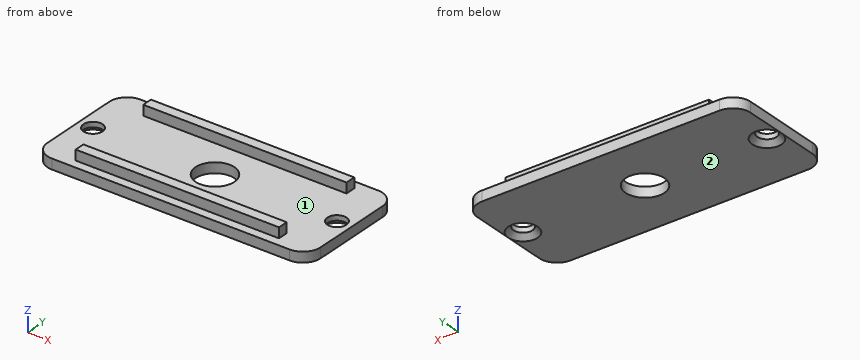
```python
from build123d import *

# Parameters (mm, degrees)
F1_DEPTH = 2
F2_R     = 1.875
F3_DEPTH = 2.001
F4_SIZE  = 0.99999
F5_W     = 40
F5_H     = 2
F6_DEPTH = 2
F7_R     = 3.81
F8_DEPTH = 2.001


# Not quite as in the source:
# - a fillet or chamfer is up to 0.001 mm smaller than in the source, because OpenCascade refuses the exact size


with BuildPart() as f1:
    # F0 (on Top) → F1 (new body)
    with BuildSketch(Plane.XY):
        with BuildLine():
            ThreePointArc((26.875, 8), (25.8498737342, 10.4748737342), (23.375, 11.5))
            Line((23.375, 11.5), (-23.375, 11.5))
            ThreePointArc((-23.375, 11.5), (-25.8498737342, 10.4748737342), (-26.875, 8))
            Line((-26.875, 8), (-26.875, -8))
            ThreePointArc((-26.875, -8), (-25.8498737342, -10.4748737342), (-23.375, -11.5))
            Line((-23.375, -11.5), (23.375, -11.5))
            ThreePointArc((23.375, -11.5), (25.8498737342, -10.4748737342), (26.875, -8))
            Line((26.875, -8), (26.875, 8))
        make_face()
    extrude(amount=F1_DEPTH)

    # F2 (on face) → F3 (cut, through all)
    with BuildSketch(Plane.XY.offset(2)):
        with Locations((-24, 0)):
            Circle(F2_R)
        with Locations((24, 0)):
            Circle(F2_R)
    extrude(amount=-F3_DEPTH, mode=Mode.SUBTRACT)

    # F4 (size 1 in the source; OpenCascade refuses exactly that, so slightly less here)
    f4_edges = [f1.edges().sort_by_distance(p)[0] for p in [
        (-25.875, 0, 0),
        (22.125, 0, 0),
    ]]
    chamfer(f4_edges, length=F4_SIZE)

    # F5 (on face) → F6 (join)
    with BuildSketch(Plane.XY.offset(2)):
        with Locations((0, 8.75)):
            Rectangle(F5_W, F5_H)
        with Locations((0, -8.75)):
            Rectangle(F5_W, F5_H)
    extrude(amount=F6_DEPTH)

    # F7 (on face) → F8 (cut, through all)
    with BuildSketch(Plane.XY.offset(2)):
        Circle(F7_R)
    extrude(amount=-F8_DEPTH, mode=Mode.SUBTRACT)


solid = f1.part
```
For this review, take the finished solid that the model builds, in its own axes (mm). Face numbers are marked on the shaded views. Round coordinates to 2 decimals unless told otherwise and drop trailing zeros. Loops run counter-clockwise (first coordinate to the right, second up) from the corner with the lowest first, then second, coordinate; pieces in that order, holes last.
(1) We need section C-C (x = -19). Give the boundary of the cut face in (y, z).
Returned:
outline: (-11.5, 0) - (11.5, 0) - (11.5, 2) - (9.75, 2) - (9.75, 4) - (7.75, 4) - (7.75, 2) - (-7.75, 2) - (-7.75, 4) - (-9.75, 4) - (-9.75, 2) - (-11.5, 2) - close
(2) We need section D-D (x = 24). Give the boundary of the cut face in (y, z) (3 decimals), plus the area to 3 significant figures.
Returned:
outline: (-11.444, 0) - (-2.875, 0) - (-1.875, 1) - (-1.875, 2) - (-11.444, 2) - close; (1.875, 1) - (2.875, 0) - (11.444, 0) - (11.444, 2) - (1.875, 2) - close
area: 37.3 mm2
(3) Mouldability with a two-part tool opening along Y and no side actions: class the marked faces 1 and 2 as released by +Y, released by -Y, zero draft, split by the parting line, or undercut.
Returned:
face 1: undercut
face 2: zero draft
(4) We need section B-B (x = 0). Give the boundary of the cut face in (y, z), plus the area to 3 significant figures.
Returned:
outline: (-11.5, 0) - (-3.81, 0) - (-3.81, 2) - (-7.75, 2) - (-7.75, 4) - (-9.75, 4) - (-9.75, 2) - (-11.5, 2) - close; (3.81, 0) - (11.5, 0) - (11.5, 2) - (9.75, 2) - (9.75, 4) - (7.75, 4) - (7.75, 2) - (3.81, 2) - close
area: 38.8 mm2
(5) Clearance check with flat-ended pins moving along their axes: P1, Ø1, axis at y = -9, z = 3, coming from the +X side; P2, Ø1.6, axis at x = -5.5, z = 3, coming from the +Y side; P3, Ø10, axis at x = 0, y = 0, coming from the +Z side. State where each tip first meets the part, or that it passes through.
Returned:
P1: stops at x = 20
P2: stops at y = 9.75
P3: stops at z = 2
(6) Wall thickness on line 1 along Z through (x, y) = (-23, 8.5); line 2 along Y through (x, z) = (-24, 1.3) (3 decimals); line 3 along X through (y, z) = (9.5, 1.3): over which ranges is each line inside the solid? List them lowest first.
Returned:
line 1: z = 0 to 2
line 2: y = -11.444 to -1.875, 1.875 to 11.444
line 3: x = -26.54 to 26.54
(7) We need section A-A (y = 0). State how many separate pieces and enclosed holes the cut face has, plus the area to 3 significant figures.
Returned:
separate pieces: 4
enclosed holes: 0
area: 75.3 mm2
